Geometry check sheet. Reference: the model listing, model coordinates, mm. A direction names the side the tool comes from. Give positions to 0.01 mm unless a question says otherwise; leave off trailing zeros. Order: outer loops, then holes, each group sorted by start corner. A loop starts at its lowest first (then second) coordinate and runs counter-clockwise, first axis right, second up.
Autodesk Inventor part; units mm, degrees
ref_plane "YZ Plane" through (0, 0, 0) normal (1, 0, 0) x (0, 1, 0)
ref_plane "XZ Plane" through (0, 0, 0) normal (0, 1, 0) x (-1, 0, 0)
ref_plane "XY Plane" through (0, 0, 0) normal (0, 0, 1) x (1, 0, 0)
sketch "Sketch1" plane through (0, 0, 0) normal (0, 0, 1) x (1, 0, 0)
  line L0 (13.5206, 26.4904) -> (14.8206, 26.4904)
  line L1 (14.8206, 26.4904) -> (14.8206, 25.1904)
  line L2 (14.8206, 25.1904) -> (16.5206, 25.1904)
  line L3 (16.5206, -8.8096) -> (14.8206, -8.8096)
  line L4 (14.8206, -8.8096) -> (14.8206, -10.1096)
  line L5 (14.8206, -10.1096) -> (13.5206, -10.1096)
  line L6 (16.5206, 25.1904) -> (16.5206, -8.8096)
  line L7 (13.5206, 25.1904) -> (14.8206, 25.1904)
  line L8 (14.8206, -8.8096) -> (13.5206, -8.8096)
  line L9 (13.5206, 26.4904) -> (13.5206, -10.1096)
  dimension "d2" = 1.3
  dimension "d15" = 3
  dimension "d16" = 1.3
  dimension "d17" = 1.3
  dimension "d18" = 1.3
  dimension "d19" = 34
  dimension "d20" = 36.6
  dimension "d21" = 1.7
extrude "Extrusion1" add sketch "Sketch1" along normal blind 60
extrude "Extrusion2" add sketch "Sketch1" against normal blind 5 contours L0 L1 L7 L9 | L8 L4 L5 L9
fillet "Fillet2" radius 1 2 edges at (14.1706, 26.4904, 60) (14.1706, -10.1096, 60)
fillet "Fillet3" radius 2 1 edges at (16.5206, 8.1904, 60)
properties part number "upper cover_3DPrint"
Item 1: Scan lines: L1, parallel to Z at x = 14.55, y = 24.5; L2, parallel to Y at x = 16.05, z = 14; L3, parallel to X at y = 25.5, z = 57. Record each from-to range of solid material in increasing order.
Reported:
L1: z = 0 to 60
L2: y = -8.81 to 25.19
L3: x = 13.52 to 14.82
Item 2: Draft check along Y on faces 1 (the cylindrical face through (15.92, 8.44, 59.43)), 2 (the flat face through (15, 8, 0)), 3 (the flat face through (14, 25.19, -2)), 4 (the flat face through (16, 25.19, 30)). Enter one of: released by +Y, released by -Y, zero draft, split by the parting line, or undercut.
Reported:
face 1: zero draft
face 2: undercut
face 3: undercut
face 4: released by +Y
Item 3: Sectioned sample at B-B (y = 15.5). Enter the section's corners in (x, z).
Reported:
outline: (13.52, 0) - (16.52, 0) - (16.52, 58) arc R2 ccw to (14.52, 60) - (13.52, 60) - close
Item 4: Gauge pin test, flat ends, axial feed: pin 1 (1 mm diameter, centred on y = 26, z = 33.5, fed in from +X); pin 2 (1.4 mm diameter, centred on x = 16, z = 34.5, fed in from -Y); pin 3 (0.9 mm diameter, centred on x = 15.5, z = 24, fed in from +Y). Record the tip position at first contact, or that the pin passes through.
Reported:
pin 1: stops at x = 14.82
pin 2: stops at y = -8.81
pin 3: stops at y = 25.19
Item 5: Sectioned sample at A-A (z = 31). Enter the section's corners in (x, y), and give its area (3 significant figures).
Reported:
outline: (13.52, -10.11) - (14.82, -10.11) - (14.82, -8.81) - (16.52, -8.81) - (16.52, 25.19) - (14.82, 25.19) - (14.82, 26.49) - (13.52, 26.49) - close
area: 105 mm2
Item 6: Set-up check for faces 5 (the flat face through (14.821, 26, 27)), 6 (the flat face through (14, -8.81, -2)), 7 (the flat face through (14.821, -9, 27)): record each of +Z, -Z, +X, -X, +Y, -Y from which the full face is reachable in a straight line by a thin tool's end or side.
Reported:
face 5: +Z, -Z, +X, +Y
face 6: -Z, +X, -X
face 7: +Z, -Z, +X, -Y
Item 7: Sectioned sample at C-C (x = 15.45). Enter the section's corners in (y, z).
Reported:
outline: (-8.81, 0) - (25.19, 0) - (25.19, 59.77) - (-8.81, 59.77) - close
